Geometry: final body of the model. Coordinates: model frame, mm. Face numbers are marked on the shaded views. A direction names the side the tool comes from. Round coordinates to 2 decimals unless told otherwise and drop trailing zeros. Loops run counter-clockwise (first coordinate to the right, second up) from the corner with the lowest first, then second, coordinate; pieces in that order, holes last. Notation, with made-up numbers: (77.5, 80.5) - (111.5, 80.5) arc R10 cw to (111.5, 86.5) - close; hole circle Ø9 at (29.5, 88.25). An arc over 180 degrees is marked (long way). Answer in a Markdown table with one row per item. Add a question column.
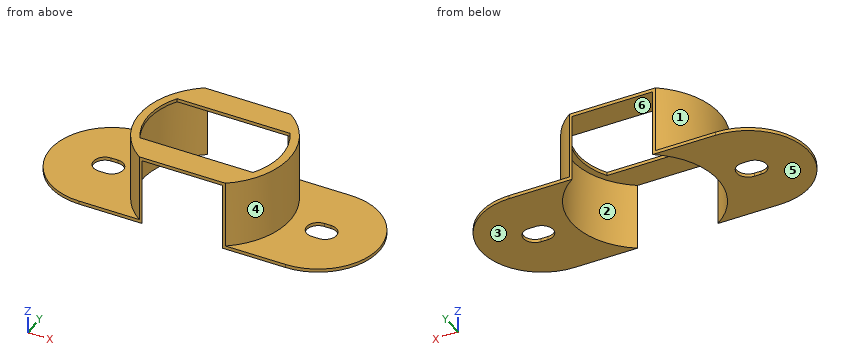
from build123d import *

# Parameters (mm, degrees)
EXTRUDE1_DEPTH     = 0.381
EXTRUDE2_DEPTH     = 7.747
CUT_EXTRUDE1_DEPTH = 7.747
CUT_EXTRUDE2_DEPTH = 9.128


with BuildPart() as part:
    # Sketch1 → Extrude1 (new body)
    with BuildSketch(Plane.XY):
        with BuildLine():
            Line((-11.8999, 6.985), (11.8999, 6.985))
            ThreePointArc((11.8999, 6.985), (18.8849, 0), (11.8999, -6.985))
            Line((11.8999, -6.985), (-11.8999, -6.985))
            ThreePointArc((-11.8999, -6.985), (-18.8849, 0), (-11.8999, 6.985))
        make_face()
        with BuildLine():
            Line((11.8999, 1.3208), (12.6873, 1.3208))
            ThreePointArc((12.6873, 1.3208), (14.0081, 0), (12.6873, -1.3208))
            Line((12.6873, -1.3208), (11.8999, -1.3208))
            ThreePointArc((11.8999, -1.3208), (10.5791, 0), (11.8999, 1.3208))
        make_face(mode=Mode.SUBTRACT)
        with BuildLine():
            Line((-12.6873, 1.3208), (-11.8999, 1.3208))
            ThreePointArc((-11.8999, 1.3208), (-10.5791, 0), (-11.8999, -1.3208))
            Line((-11.8999, -1.3208), (-12.6873, -1.3208))
            ThreePointArc((-12.6873, -1.3208), (-14.0081, 0), (-12.6873, 1.3208))
        make_face(mode=Mode.SUBTRACT)
    extrude(amount=EXTRUDE1_DEPTH)

    # Sketch2 → Extrude2 (add)
    with BuildSketch(Plane.XY.offset(0.381)):
        with BuildLine():
            Line((-4.96966108, -6.985), (4.96966108, -6.985))
            ThreePointArc((4.96966108, -6.985), (8.5725, 0), (4.96966108, 6.985))
            Line((4.96966108, 6.985), (-4.96966108, 6.985))
            ThreePointArc((-4.96966108, 6.985), (-8.5725, 0), (-4.96966108, -6.985))
        make_face()
    extrude(amount=EXTRUDE2_DEPTH)

    # Sketch3 → Cut-Extrude1 (cut)
    with BuildSketch(Plane(origin=(0, 0, 0), x_dir=(-1, 0, 0), z_dir=(0, 0, -1))):
        with BuildLine():
            Line((-4.633324832, 6.985), (4.633324832, 6.985))
            ThreePointArc((4.633324832, 6.985), (8.382, 0), (4.633324832, -6.985))
            Line((4.633324832, -6.985), (-4.633324832, -6.985))
            ThreePointArc((-4.633324832, -6.985), (-8.382, 0), (-4.633324832, 6.985))
        make_face()
    extrude(amount=-CUT_EXTRUDE1_DEPTH, mode=Mode.SUBTRACT)

    # Sketch4 → Cut-Extrude2 (cut, through all)
    with BuildSketch(Plane.XY.offset(8.128)):
        with BuildLine():
            Line((-6.508746902, 3.9624), (6.508746902, 3.9624))
            ThreePointArc((6.508746902, 3.9624), (7.62, 0), (6.508746902, -3.9624))
            Line((6.508746902, -3.9624), (-6.508746902, -3.9624))
            ThreePointArc((-6.508746902, -3.9624), (-7.62, 0), (-6.508746902, 3.9624))
        make_face()
    extrude(amount=-CUT_EXTRUDE2_DEPTH, mode=Mode.SUBTRACT)


solid = part.part
1) Section B-B, the plane y = 0. Return the cut outline in (x, z).
2) Pull-direction query (X, two-part tool) for the marked faces 1, 2 and 3; classes: pulls with the +X half, pulls with the -X half, needs draft (parallel to the pull), parting line crosses it, or undercut.
3) Section D-D, the plane y = -2.5. Return the cut outline in (x, z).
4) Reachability of the marked faces 4, 5 and 6 from +Z, -Z, +X, -X, +Y, -Y: full face, straight path, thin tool, end or side. Return the list, or none.
5) Section A-A, the plane x = -0.5. Return the cut outline in (y, z) (3 decimals), and give its area (3 significant figures).
6) Contact query for flat-ended pins moving along their axis: pin 1 Ø7 at (x, y) = (15, 1.5) entering from +Z; pin 2 Ø8 at (x, y) = (4.5, 4.5) entering from -Z; pin 3 Ø3 at (y, z) = (5.5, 7) entering from +X; pin 4 Ø1.5 at (x, z) = (8, 3) entering from +Y. Output: stop coordinate, or through.
7) Material intervals for line 1 along X through (y, z) = (0.25, 1.5); line 2 along Z through (x, y) = (-3.5, 5); line 3 along X through (y, z) = (-6.5, 1.5), sorted ascending. Write a range as from..to.
Evaluation:
| question | item | result |
|---|---|---|
| 1 | outline | (-18.88, 0) - (-14.01, 0) - (-14.01, 0.38) - (-18.88, 0.38) - close; (-10.58, 0) - (-8.38, 0) - (-8.38, 7.75) - (-7.62, 7.75) - (-7.62, 8.13) - (-8.57, 8.13) - (-8.57, 0.38) - (-10.58, 0.38) - close; (7.62, 7.75) - (8.38, 7.75) - (8.38, 0) - (10.58, 0) - (10.58, 0.38) - (8.57, 0.38) - (8.57, 8.13) - (7.62, 8.13) - close; (14.01, 0) - (18.88, 0) - (18.88, 0.38) - (14.01, 0.38) - close |
| 2 | face 1 | pulls with the -X half |
| 2 | face 2 | undercut |
| 2 | face 3 | needs draft |
| 3 | outline | (-18.42, 0) - (-8, 0) - (-8, 7.75) - (-7.2, 7.75) - (-7.2, 8.13) - (-8.2, 8.13) - (-8.2, 0.38) - (-18.42, 0.38) - close; (7.2, 7.75) - (8, 7.75) - (8, 0) - (18.42, 0) - (18.42, 0.38) - (8.2, 0.38) - (8.2, 8.13) - (7.2, 8.13) - close |
| 4 | face 4 | +Z, +X |
| 4 | face 5 | -Z, +X, -X, +Y, -Y |
| 4 | face 6 | -Z |
| 5 | outline | (-6.985, 7.747) - (-3.962, 7.747) - (-3.962, 8.128) - (-6.985, 8.128) - close; (3.962, 7.747) - (6.985, 7.747) - (6.985, 8.128) - (3.962, 8.128) - close |
| 5 | area | 2.30 mm² |
| 6 | pin 1 | stops at z = 0.38 |
| 6 | pin 2 | stops at z = 0 |
| 6 | pin 3 | stops at x = 7.58 |
| 6 | pin 4 | stops at y = 4.57 |
| 7 | line 1 | x = -8.57..-8.38, 8.38..8.57 |
| 7 | line 2 | z = 7.75..8.13 |
| 7 | line 3 | x = -5.59..-5.29, 5.29..5.59 |
